Here's how the part is built. I have some questions about the finished solid (model axes, mm). Face numbers are marked on the shaded views. Give positions to 0.01 mm unless a question says otherwise; leave off trailing zeros. Loops run counter-clockwise (first coordinate to the right, second up) from the corner with the lowest first, then second, coordinate; pieces in that order, holes last.
Q1. Suppose I cut it at C-C (z = 13). List the corners of the cut face in (x, y) for me.
Q2. Suppose I cut it at A-A (y = 0). List the corners of the cut face in (x, z) for me, and give its area (3 significant figures).
Q3. I'm going to push flat-ended pins straight in: P1, Ø10, axis at y = 0.5, z = -9, coming from the +X side; P2, Ø6, axis at x = 8.5, z = 4.5, coming from the -Y side; P3, Ø2, axis at x = 9.5, z = -3.5, coming from the +Y side; P4, Ø4, axis at x = -10, y = -3.5, coming from the +Z side. Where does each tip first touch, or does it pass through?
Q4. Thinking about a two-plate mould opening in X: for the marked faces 1, 2 and 3, which applies, pulls with the +X half, pulls with the -X half, needs draft (parallel to the pull), parting line crosses it, or undercut?
Q5. I need wall thicknesses on probe 1 along Y at (x, z) = (0, 10.5); probe 2 along X at (y, z) = (5.5, 20); probe 3 along Y at (x, z) = (-11, 12). Which ranges of each line are inside material? Lowest first, please.
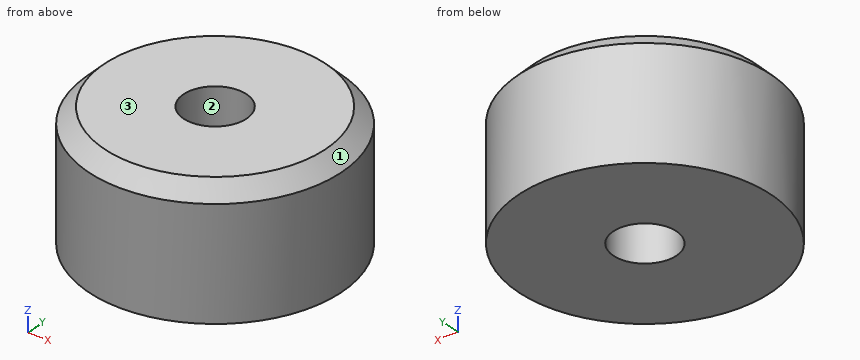
```python
from build123d import *

# Parameters (mm, degrees)
F0_R     = 50.8
F0_R_2   = 12.7
F1_DEPTH = 25.4
F2_SIZE  = 6.35
F3_DEPTH = 25.4


with BuildPart() as f1:
    # F0 (on Top) → F1 (new body)
    with BuildSketch(Plane.XY):
        Circle(F0_R)
        Circle(F0_R_2, mode=Mode.SUBTRACT)
    extrude(amount=F1_DEPTH)

    # F2
    f2_edges = [f1.edges().sort_by_distance(p)[0] for p in [
        (-50.8, 0, 25.4),
    ]]
    chamfer(f2_edges, length=F2_SIZE)

    # F0 (on Top) → F3 (join)
    with BuildSketch(Plane.XY):
        Circle(F0_R)
        Circle(F0_R_2, mode=Mode.SUBTRACT)
    extrude(amount=-F3_DEPTH)


solid = f1.part
```
Solutions:
1. outline: circle Ø101.6 at (0, 0); hole circle Ø25.4 at (0, 0)
2. outline: (-50.8, -25.4) - (-12.7, -25.4) - (-12.7, 25.4) - (-44.45, 25.4) - (-50.8, 19.05) - close; (12.7, -25.4) - (50.8, -25.4) - (50.8, 19.05) - (44.45, 25.4) - (12.7, 25.4) - close
2. area: 3,830 mm2
3. P1: stops at x = 50.8
3. P2: stops at y = -50.5
3. P3: stops at y = 50.08
3. P4: passes through
4. face 1: parting line crosses it
4. face 2: undercut
4. face 3: needs draft
5. probe 1: y = -50.8 to -12.7, 12.7 to 50.8
5. probe 2: x = -49.55 to -11.45, 11.45 to 49.55
5. probe 3: y = -49.59 to -6.35, 6.35 to 49.59
